Input: part model. Units: mm. Frame: model coordinates. Face numbers are marked on the shaded views. A direction names the side the tool comes from. Coordinates: 2 decimals unless noted, no trailing zeros. Order: outer loops, then holes, each group sorted by start corner. A loop starts at its lowest first (then second) coordinate and runs counter-clockwise, first axis right, second up. Notation, with made-up numbers: (-32.75, 48) -> (18.25, 48) arc R10 ccw to (18.25, 63) -> close; hole circle Ø7 at (43, 45.25). An arc over 180 degrees is marked (long way). Write each question's results on one line, items separated by ' | '.
```python
from build123d import *

# Parameters (mm, degrees)
SKETCH1_R                                           = 4.9975
BOSS_EXTRUDE1_DEPTH                                 = 4.999999995
SKETCH5_R                                           = 16.129
CUT_EXTRUDE2_DEPTH                                  = 2.032
F_5_0MM_DOWEL_HOLE1_D                               = 5
F_5_0MM_DOWEL_HOLE1_DEPTH                           = 16.51
F_5_0MM_DOWEL_HOLE1_TIP                             = 1.502151548
CSK_FOR_1_4_FLAT_HEAD_MACHINE_SCREW_100_D           = 6.5278
CSK_FOR_1_4_FLAT_HEAD_MACHINE_SCREW_100_DEPTH       = 16.51
CSK_FOR_1_4_FLAT_HEAD_MACHINE_SCREW_100_CSINK_D     = 12.8778
CSK_FOR_1_4_FLAT_HEAD_MACHINE_SCREW_100_CSINK_ANGLE = 100
CSK_FOR_1_4_FLAT_HEAD_MACHINE_SCREW_100_TIP         = 1.961148974
SKETCH26_W                                          = 9.99999999
SKETCH26_H                                          = 10.000000066
BOSS_EXTRUDE2_DEPTH                                 = 24.500000022
FILLET1_R                                           = 2.54
F_7_32_0_21875_DIAMETER_HOLE1_D                     = 5.55625
F_7_32_0_21875_DIAMETER_HOLE1_DEPTH                 = 16.51
F_7_32_0_21875_DIAMETER_HOLE1_TIP                   = 1.669265907


with BuildPart() as part:
    # Sketch1 → Boss-Extrude1 (new, symmetric)
    with BuildSketch(Plane.XY):
        with BuildLine():
            Line((-12.7, -80.01), (12.7, -80.01))
            Line((12.7, -80.01), (12.7, -23.452055347))
            ThreePointArc((12.7, -23.452055347), (0, 26.67), (-12.7, -23.452055347))
            Line((-12.7, -23.452055347), (-12.7, -80.01))
        make_face()
        Circle(SKETCH1_R, mode=Mode.SUBTRACT)
    extrude(amount=BOSS_EXTRUDE1_DEPTH, both=True)

    # Sketch5 → Cut-Extrude2 (cut)
    with BuildSketch(Plane.XY.offset(4.999999995)):
        Circle(SKETCH5_R)
    extrude(amount=-CUT_EXTRUDE2_DEPTH, mode=Mode.SUBTRACT)

    # Ø5.0mm Dowel Hole1
    with Locations(Plane(origin=(11.43, 0, -4.999999995), x_dir=(-1, 0, 0), z_dir=(0, 0, -1))):
        with Locations((0, 0), (22.86, 0)):
            Hole(F_5_0MM_DOWEL_HOLE1_D / 2, depth=F_5_0MM_DOWEL_HOLE1_DEPTH)
            with Locations((0, 0, -(F_5_0MM_DOWEL_HOLE1_DEPTH + F_5_0MM_DOWEL_HOLE1_TIP / 2))):  # 118° drill point
                Cone(0, F_5_0MM_DOWEL_HOLE1_D / 2, F_5_0MM_DOWEL_HOLE1_TIP, mode=Mode.SUBTRACT)

    # CSK for 1/4 Flat Head Machine Screw (100)1
    with Locations(Plane(origin=(0, 11.43, -4.999999995), x_dir=(-1, 0, 0), z_dir=(0, 0, -1))):
        with Locations((0, 0), (0, -22.86)):
            CounterSinkHole(CSK_FOR_1_4_FLAT_HEAD_MACHINE_SCREW_100_D / 2, CSK_FOR_1_4_FLAT_HEAD_MACHINE_SCREW_100_CSINK_D / 2, depth=CSK_FOR_1_4_FLAT_HEAD_MACHINE_SCREW_100_DEPTH, counter_sink_angle=CSK_FOR_1_4_FLAT_HEAD_MACHINE_SCREW_100_CSINK_ANGLE)
            with Locations((0, 0, -(CSK_FOR_1_4_FLAT_HEAD_MACHINE_SCREW_100_DEPTH + CSK_FOR_1_4_FLAT_HEAD_MACHINE_SCREW_100_TIP / 2))):  # 118° drill point
                Cone(0, CSK_FOR_1_4_FLAT_HEAD_MACHINE_SCREW_100_D / 2, CSK_FOR_1_4_FLAT_HEAD_MACHINE_SCREW_100_TIP, mode=Mode.SUBTRACT)

    # Sketch26 → Boss-Extrude2 (add, symmetric)
    with BuildSketch(Plane(origin=(0, 0, 0), x_dir=(0, 0, -1), z_dir=(1, 0, 0))):
        with Locations((0, -75.009999967)):
            Rectangle(SKETCH26_W, SKETCH26_H)
    extrude(amount=BOSS_EXTRUDE2_DEPTH, both=True)

    # Fillet1
    fillet1_edges = [part.edges().sort_by_distance(p)[0] for p in [
        (12.7, -23.452055347, 0),
        (12.7, -70.009999934, 0),
        (-12.7, -23.452055347, 0),
        (-12.7, -70.009999934, 0),
        (-24.500000022, -70.009999934, 0),
        (-24.500000022, -80.01, 0),
        (24.500000022, -70.009999934, 0),
        (24.500000022, -80.01, 0),
    ]]
    fillet(fillet1_edges, radius=FILLET1_R)

    # 7/32 (0.21875) Diameter Hole1
    with Locations(Plane(origin=(-18.749999584, -75.009999967, -4.999999995), x_dir=(-1, 0, 0), z_dir=(0, 0, -1))):
        with Locations((0, 0), (-12.499999892, 0), (-24.999999784, 0), (-37.499999676, 0)):
            Hole(F_7_32_0_21875_DIAMETER_HOLE1_D / 2, depth=F_7_32_0_21875_DIAMETER_HOLE1_DEPTH)
            with Locations((0, 0, -(F_7_32_0_21875_DIAMETER_HOLE1_DEPTH + F_7_32_0_21875_DIAMETER_HOLE1_TIP / 2))):  # 118° drill point
                Cone(0, F_7_32_0_21875_DIAMETER_HOLE1_D / 2, F_7_32_0_21875_DIAMETER_HOLE1_TIP, mode=Mode.SUBTRACT)


solid = part.part
```
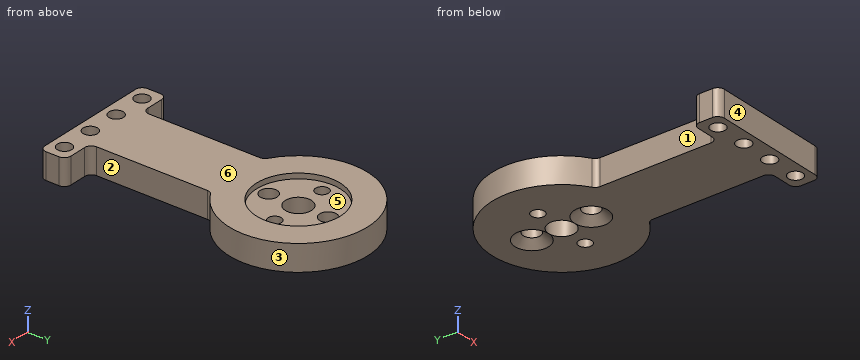
(1) Cut plane C-C, the plane y = 11.43. Return loops of the section in (x, z).
Return value:
outline: (-24.1, -5) -> (-6.44, -5) -> (-3.26, -2.34) -> (-3.26, 2.97) -> (-11.38, 2.97) -> (-11.38, 5) -> (-24.1, 5) -> close; (3.26, -2.34) -> (6.44, -5) -> (24.1, -5) -> (24.1, 5) -> (11.38, 5) -> (11.38, 2.97) -> (3.26, 2.97) -> close
(2) Cut plane A-A, the plane x = -11.43. Return loops of the section in (y, z), plus the area to 3 significant figures.
Return value:
outline: (-80.01, -5) -> (-2.5, -5) -> (-2.5, 2.97) -> (-11.38, 2.97) -> (-11.38, 5) -> (-80.01, 5) -> close; (2.5, -5) -> (24.1, -5) -> (24.1, 5) -> (11.38, 5) -> (11.38, 2.97) -> (2.5, 2.97) -> close | area: 955 mm2
(3) Cut plane D-D, the plane x = 10. Return loops of the section in (y, z), plus the area to 3 significant figures.
Return value:
outline: (-80.01, -5) -> (-2.05, -5) -> (-2.05, 2.97) -> (-12.65, 2.97) -> (-12.65, 5) -> (-80.01, 5) -> close; (2.05, -5) -> (24.72, -5) -> (24.72, 5) -> (12.65, 5) -> (12.65, 2.97) -> (2.05, 2.97) -> close | area: 963 mm2
(4) Reachability of the marked faces 1, 2 and 3 from +Z, -Z, +X, -X, +Y, -Y: full face, straight path, thin tool, end or side. Return the list, or none.
Return value:
face 1: +Z, -Z, -X | face 2: +Z, -Z, +X | face 3: +Z, -Z
(5) Cut plane B-B, the plane x = 18.75. Return loops of the section in (y, z), plus the area to 3 significant figures.
Return value:
outline: (-80.01, -5) -> (-77.79, -5) -> (-77.79, 5) -> (-80.01, 5) -> close; (-72.23, -5) -> (-70.01, -5) -> (-70.01, 5) -> (-72.23, 5) -> close; (-18.97, -5) -> (18.97, -5) -> (18.97, 5) -> (-18.97, 5) -> close | area: 424 mm2
(6) Pin query (flat end, axial travel): P1, Ø5, axis at y = -27.5, z = 0, coming from the +X side; P2, Ø3.5, axis at x = 19.5, z = -0.5, coming from the +Y side; P3, Ø2, axis at x = -19, z = 0, coming from the +Y side. Return the tip coordinate at first contact, or that it passes through.
Return value:
P1: x = 12.7 | P2: y = 19.91 | P3: y = 19.68
(7) Mould query, pull axis Y, two halves, no side actions, for the marked faces 4, 5 and 6. Classes: +Y half, -Y half, draft (parallel to the pull), parting line (faces both ways), or undercut.
Return value:
face 4: -Y half | face 5: undercut | face 6: draft
(8) Line query: line 1 along Y through (x, z) = (0, 0.9); line 2 along X through (y, z) = (-75, 1.5); line 3 along Y through (x, z) = (0, 3.9). Output: solid intervals per line, ascending. Write a range as from..to.
Return value:
line 1: -80.01..-14.69, -8.17..-5, 5..8.17, 14.69..26.67 | line 2: -24.5..-21.53, -15.97..-9.03, -3.47..3.47, 9.03..15.97, 21.53..24.5 | line 3: -80.01..-16.13, 16.13..26.67
